Geometry: final body of the model. Coordinates: model frame, mm. Face numbers are marked on the shaded views. A direction names the side the tool comes from. Give positions to 0.01 mm unless a question says otherwise; leave off trailing zeros. Loops run counter-clockwise (first coordinate to the right, second up) from the corner with the lowest first, then second, coordinate; pieces in that order, holes last.
```python
from build123d import *

# Parameters (mm, degrees)
CROQUIS1_W              = 1800
CROQUIS1_H              = 610
SALIENTE_EXTRUIR1_DEPTH = 600
CROQUIS2_W              = 40.721486725
CROQUIS2_H              = 600
CROQUIS2_W_2            = 34.613400616
CORTAR_EXTRUIR1_DEPTH   = 2
CROQUIS3_W              = 490.887470824
CROQUIS3_H              = 496.465737538
CROQUIS3_W_2            = 468.574403969
CROQUIS3_W_3            = 429.526536971
CORTAR_EXTRUIR2_DEPTH   = 52
CROQUIS4_R              = 33.469600283
CROQUIS4_R_2            = 36.25873364
CROQUIS4_R_3            = 37.420150707
CORTAR_EXTRUIR3_DEPTH   = 52
MATRIZL1_COUNT          = 3
MATRIZL1_PITCH          = 600
SALIENTE_EXTRUIR2_DEPTH = 666
CROQUIS6_W              = 1800
CROQUIS6_H              = 610
SALIENTE_EXTRUIR3_DEPTH = 300


with BuildPart() as part:
    # Croquis1 → Saliente-Extruir1 (new body)
    with BuildSketch(Plane(origin=(0, 0, 0), x_dir=(1, 0, 0), z_dir=(0, 1, 0))):
        Rectangle(CROQUIS1_W, CROQUIS1_H)
    extrude(amount=SALIENTE_EXTRUIR1_DEPTH)

    # Croquis2 → Cortar-Extruir1 (cut)
    with BuildSketch(Plane.XY.offset(305)):
        with Locations((-274.287558023, 300)):
            Rectangle(CROQUIS2_W, CROQUIS2_H)
        with Locations((327.607420408, 300)):
            Rectangle(CROQUIS2_W_2, CROQUIS2_H)
    extrude(amount=-CORTAR_EXTRUIR1_DEPTH, mode=Mode.SUBTRACT)

    # Croquis3 → Cortar-Extruir2 (cut)
    with BuildSketch(Plane.XY.offset(305)):
        with Locations((-568.983204819, 309.761966749)):
            Rectangle(CROQUIS3_W, CROQUIS3_H)
        with Locations((30.680466927, 309.761966749)):
            Rectangle(CROQUIS3_W_2, CROQUIS3_H)
        with Locations((591.296271675, 309.761966749)):
            Rectangle(CROQUIS3_W_3, CROQUIS3_H)
    extrude(amount=-CORTAR_EXTRUIR2_DEPTH, mode=Mode.SUBTRACT)

    # Croquis4 → Cortar-Extruir3 (cut)
    with BuildSketch(Plane.XY.offset(253)):
        with Locations((-738.199956824, 312.551100106)):
            Circle(CROQUIS4_R)
        with Locations((-602.642790268, 312.551100106)):
            Circle(CROQUIS4_R_2)
        with Locations((-430.405449232, 312.551100106)):
            Circle(CROQUIS4_R_3)
    cortar_extruir3 = extrude(amount=-CORTAR_EXTRUIR3_DEPTH, mode=Mode.SUBTRACT)

    # MatrizL1: Cortar-Extruir3 ×3
    with Locations(*[(i * MATRIZL1_PITCH, 0, 0) for i in range(1, MATRIZL1_COUNT)]):
        add(cortar_extruir3, mode=Mode.SUBTRACT)

    # Croquis5 → Saliente-Extruir2 (add)
    with BuildSketch(Plane(origin=(0, 600, 0), x_dir=(1, 0, 0), z_dir=(0, 1, 0))):
        Polygon((900, -305), (880, -305), (880, -285), (880, 285), (-880, 285), (-880, -285), (-880, -305), (-900, -305), (-900, 305), (900, 305), align=None)
    extrude(amount=SALIENTE_EXTRUIR2_DEPTH)

    # Croquis6 → Saliente-Extruir3 (add)
    with BuildSketch(Plane(origin=(0, 1266, 0), x_dir=(1, 0, 0), z_dir=(0, 1, 0))):
        Rectangle(CROQUIS6_W, CROQUIS6_H)
    extrude(amount=SALIENTE_EXTRUIR3_DEPTH)


solid = part.part
```
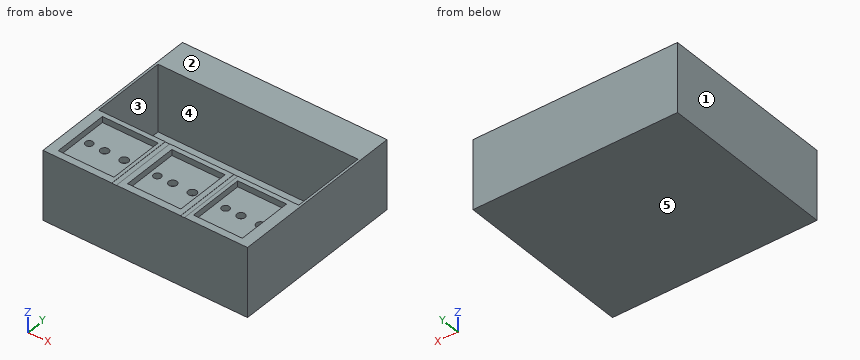
Q1. Reachability of the marked faces 4 and 5 from +Z, -Z, +X, -X, +Y, -Y: full face, straight path, thin tool, end or side. Return the list, or none.
Q2. Mould query, pull axis X, two halves, no side actions, for the marked faces 1, 2 and 3. Classes: +X half, -X half, draft (parallel to the pull), parting line (faces both ways), or undercut.
Q3. Pin query (flat end, axial travel): pin 1 Ø5 at (x, y) = (631.5, 854) entering from +Z; pin 2 Ø5 at (x, z) = (-707, -205) entering from -Y; pin 3 Ø6 at (x, y) = (-286.5, 470.5) entering from +Z; pin 4 Ø20 at (x, y) = (-751, 318.5) entering from +Z. Return the tip coordinate at first contact, or that it passes through.
Q4. Section query B-B, the plane z = -1. Return loops of the section in (x, y), and give its area (3 significant figures).
Q5. Material intervals for probe 1 along X at (y, z) = (845.5, 35); probe 2 along Y at (x, z) = (-328, -205); probe 3 along Z at (x, y) = (558, 1053), sorted ascending.
Q6. Section query D-D, the plane x = -534. Return loops of the section in (y, z).
Q7. Section query C-C, the plane y = 1166.5. Return loops of the section in (x, z).
Q8. Section query A-A, the plane x = -230. Return loops of the section in (y, z), and give its area (3 significant figures).
Resolved:
1. face 4: +Z
1. face 5: -Z, +X, -X, +Y, -Y
2. face 1: -X half
2. face 2: draft
2. face 3: undercut
3. pin 1: stops at z = -285
3. pin 2: stops at y = 0
3. pin 3: stops at z = 303
3. pin 4: stops at z = 201
4. outline: (-900, 0) - (900, 0) - (900, 1566) - (-900, 1566) - close; hole (-880, 600) - (880, 600) - (880, 1266) - (-880, 1266) - close
4. area: 1,650,000 mm2
5. probe 1: x = -900 to -880, 880 to 900
5. probe 2: y = 0 to 600, 1266 to 1566
5. probe 3: z = -305 to -285
6. outline: (0, -305) - (1566, -305) - (1566, 305) - (1266, 305) - (1266, -285) - (600, -285) - (600, 305) - (557.99, 305) - (557.99, 253) - (61.53, 253) - (61.53, 305) - (0, 305) - close
7. outline: (-900, -305) - (900, -305) - (900, 305) - (880, 305) - (880, -285) - (-880, -285) - (-880, 305) - (-900, 305) - close
8. outline: (0, -305) - (1566, -305) - (1566, 305) - (1266, 305) - (1266, -285) - (600, -285) - (600, 305) - (0, 305) - close
8. area: 562,000 mm2
